Autodesk Inventor part; units mm, degrees
ref_plane "YZ Plane" through (0, 0, 0) normal (1, 0, 0) x (0, 1, 0)
ref_plane "XZ Plane" through (0, 0, 0) normal (0, 1, 0) x (-1, 0, 0)
ref_plane "XY Plane" through (0, 0, 0) normal (0, 0, 1) x (1, 0, 0)
sketch "Sketch9" plane through (0, 0, 0) normal (0, 0, 1) x (1, 0, 0)
  circle A0 centre (0, 0) radius 4.125 construction
  circle A1 centre (0, 0) radius 16.5
  circle A2 centre (11, 0) radius 2.4
  circle A3 centre (5.5, 9.5263) radius 2.4
  circle A4 centre (-5.5, 9.5263) radius 2.4
  line L0 (-3.4894, 2.2) -> (3.4894, 2.2)
  arc A5 (-3.4894, 2.2) -> (3.4894, 2.2) centre (0, 0) ccw
  circle A6 centre (-11, 0) radius 2.4
  circle A7 centre (-5.5, -9.5263) radius 2.4
  circle A8 centre (5.5, -9.5263) radius 2.4
  dimension "d25" = 8.25
  dimension "d26" = 33
  dimension "d27" = 4.8
  dimension "d31" = 360
  dimension "d33" = 2.2
  dimension "d36" = 11
extrude "Extrusion8" add sketch "Sketch9" along normal blind 12.7
sketch "Sketch10" plane through (-3.4894, 2.2, 0) normal (0, -1, 0) x (1, 0, 0)
  line L0 (6.9787, 0) -> (0, 0)
  line L1 (6.9787, 0) -> (6.9787, 12.7)
  line L2 (0, 12.7) -> (6.9787, 12.7)
  line L3 (0, 0) -> (0, 12.7)
  circle A0 centre (3.4894, 6.35) radius 2.5
  point P0 (3.4894, 0)
  point P1 (3.4894, 12.7)
  point P2 (0, 6.35)
  dimension "d37" = 5
extrude "Extrusion9" cut sketch "Sketch10" against normal through all contours A0
sketch "Sketch11" plane through (0, 0, 12.7) normal (0, 0, 1) x (1, 0, 0)
  line L0 (4.9483, 5.1999) -> (6.9612, 5.1999)
  line L1 (6.9612, 5.1999) -> (6.9612, 2.6)
  line L2 (6.9612, 2.6) -> (4.9483, 2.6)
  line L3 (4.9483, 2.6) -> (4.9483, 5.1999)
  point P0 (0, 0)
extrude "Extrusion10" cut sketch "Sketch11" against normal blind 0.1
properties part number "AA057" material "Aluminum 6061"
For this review, take the finished solid that the model builds, in its own axes (mm). A direction names the side the tool comes from. Give positions to 0.01 mm unless a question says otherwise; leave off trailing zeros. Loops run counter-clockwise (first coordinate to the right, second up) from the corner with the lowest first, then second, coordinate; pieces in that order, holes last. Notation, with made-up numbers: M 41.25,71.25 L 82.25,71.25 A13 cw 82.25,76.25 Z; hole C 69,47.5 d2. An arc over 180 degrees is marked long. Answer as a JSON object with one key per item and string values. Group by question number.
Q1. For probe 1 along X at (y, z) = (9.5, 1.75); probe 2 along X at (y, z) = (11.5, 9.75); probe 3 along Z at (x, y) = (0, 13.75), list the stretches that pass through material, from the lowest coordinate up. Write a range as [from, to].
Q2. Tool access review of faces 1 (the flat face through (-2.4, 2.2, 4.8)), 2 (the cylindrical face through (-0.33, 9.25, 8.83)), 3 (the flat face through (0, 4, 0)): name each direction out of +Z, -Z, +X, -X, +Y, -Y from which nothing blocks a thin tool from reaching the whole face with its end or side.
Q3. Add section D-D on y = 0. Give the boundary of the cut face in (x, z), and give its area (3 significant figures).
Q4. Add section C-C on z = 3. Give the boundary of the cut face in (x, y).
Q5. Add section B-B on y = 8. Give the boundary of the cut face in (x, z), and give its area (3 significant figures).
Q6. Mouldability with a two-part tool opening along X and no side actions: class faces 4 (the flat face through (0, 4, 12.7)), 5 (the cylindrical face through (15.24, 6.32, 6.26)), 6 (the flat face through (6, 4, 12.6)) as +X half, -X half, draft (parallel to the pull), parting line (faces both ways), or undercut.
Q7. Add section A-A on x = 0. Give the boundary of the cut face in (y, z), and give its area (3 significant figures).
Q8. Insertion check: P1, Ø3, axis at x = -11, y = 0, coming from the +Z side; P2, Ø4, axis at x = 10.5, z = 5, coming from the -Y side; P3, Ø1, axis at x = -7, z = 10, coming from the -Y side; P4, Ø6, axis at y = -5.5, z = 4.5, coming from the +X side. Each pin has a flat end and moves straight along its axis. Give the tip position at first contact, or say it passes through.
Checked values:
{
 "1": {"probe 1": "[-13.49, -7.9], [-3.1, 3.1], [7.9, 13.49]", "probe 2": "[-11.83, -6.87], [-4.13, 4.13], [6.87, 11.83]", "probe 3": "[0, 3.85], [8.85, 12.7]"},
 "2": {"face 1": "+Z, -Z", "face 2": "+Y", "face 3": "-Z, +X, -X, +Y, -Y"},
 "3": {"outline": "M -16.5,0 L -13.4,0 L -13.4,12.7 L -16.5,12.7 Z; M -8.6,0 L -4.13,0 L -4.13,12.7 L -8.6,12.7 Z; M 4.13,0 L 8.6,0 L 8.6,12.7 L 4.13,12.7 Z; M 13.4,0 L 16.5,0 L 16.5,12.7 L 13.4,12.7 Z", "area": "192 mm²"},
 "4": {"outline": "C 0,0 d33; hole C -11,0 d4.8; hole C -5.5,-9.53 d4.8; hole C -5.5,9.53 d4.8; hole M -3.49,2.2 A4.13 ccw long 3.49,2.2 Z; hole C 5.5,-9.53 d4.8; hole C 5.5,9.53 d4.8; hole C 11,0 d4.8"},
 "5": {"outline": "M -14.43,0 L -7.35,0 L -7.35,12.7 L -14.43,12.7 Z; M -3.65,0 L 3.65,0 L 3.65,12.7 L -3.65,12.7 Z; M 7.35,0 L 14.43,0 L 14.43,12.7 L 7.35,12.7 Z; hole C 0,6.35 d5", "area": "253 mm²"},
 "6": {"face 4": "draft", "face 5": "parting line", "face 6": "undercut"},
 "7": {"outline": "M -16.5,0 L -4.13,0 L -4.13,12.7 L -16.5,12.7 Z; M 2.2,0 L 16.5,0 L 16.5,3.85 L 2.2,3.85 Z; M 2.2,8.85 L 16.5,8.85 L 16.5,12.7 L 2.2,12.7 Z", "area": "267 mm²"},
 "8": {"P1": "through", "P2": "y = -14.14", "P3": "y = -15.17", "P4": "x = 16.31"}
}
